from build123d import *

# Parameters (mm, degrees)
F0_R     = 6.35
F0_R_2   = 5.588
F1_DEPTH = 6.35
F0_R_3   = 0.638783
F0_R_4   = 1.905
F2_DEPTH = 5.969


with BuildPart() as f1:
    # F0 (on Top) → F1 (new body, symmetric)
    with BuildSketch(Plane.XY):
        Circle(F0_R)
        Circle(F0_R_2, mode=Mode.SUBTRACT)
    extrude(amount=F1_DEPTH, both=True)

    # F0 (on Top) → F2 (join, symmetric)
    with BuildSketch(Plane.XY):
        Circle(F0_R_2)
        with Locations((-2.271086, -3.125882)):
            Circle(F0_R_3, mode=Mode.SUBTRACT)
        Circle(F0_R_4, mode=Mode.SUBTRACT)
        with Locations((2.271086, -3.125882)):
            Circle(F0_R_3, mode=Mode.SUBTRACT)
        with Locations((-3.674694, 1.193981)):
            Circle(F0_R_3, mode=Mode.SUBTRACT)
        with Locations((0, 3.863802)):
            Circle(F0_R_3, mode=Mode.SUBTRACT)
        with Locations((3.674694, 1.193981)):
            Circle(F0_R_3, mode=Mode.SUBTRACT)
    extrude(amount=F2_DEPTH, both=True)


solid = f1.part
Verification items for the finished model (mm, model axes). A direction names the side the tool comes from. Coordinates: 2 decimals unless noted, no trailing zeros. Order: outer loops, then holes, each group sorted by start corner. A loop starts at its lowest first (then second) coordinate and runs counter-clockwise, first axis right, second up. Notation, with made-up numbers: M 85.25,-6 L 94.25,-6 A10 cw 94.25,1 Z; hole C 37.5,22 d1. An arc over 180 degrees is marked long. One line per item, written item: value. Start each with the question number.
Item 1: Mould release check, pull along X, two halves, no side actions. Record for faces 1 (the cylindrical face through (-1.38, -6.2, 0.09)), 2 (the cylindrical face through (2.88, -2.93, -0.08)), 3 (the flat face through (0, -6, 6.35)): released by +X, released by -X, zero draft, split by the parting line, or undercut.
Item 2: Gauge pin test, flat ends, axial feed: pin 1 (1.5 mm diameter, centred on y = -2.5, z = 2, fed in from -X); pin 2 (1.5 mm diameter, centred on x = -4, z = -2.5, fed in from +Y); pin 3 (2 mm diameter, centred on y = -1.5, z = 2, fed in from +X); pin 4 (4 mm diameter, centred on x = -5, y = 1.5, fed in from +Z). Record the tip position at first contact, or that the pin passes through.
Item 3: Scan lines: probe 1 along X at (y, z) = (1, 0.25); probe 2 along Y at (x, z) = (0, 6); probe 3 along Z at (x, y) = (1.5, -1.5). Record each from-to range of solid material in increasing order.
Item 4: Sectioned sample at B-B (x = 0). Enter the section's corners in (y, z) (3 decimals).
Item 5: Access from +Z, -Z, +X, -X, +Y, -Y to the whole of each face (thin tool, end or side, straight path). Record for faces 4 (the flat face through (2.4, 0.1, -5.969)), 5 (the flat face through (2.4, 0.1, 5.969)), 6 (the cylindrical face through (-3.085, 0.949, -0.084)).
Item 6: Sectioned sample at D-D (z = 3). Enter the section's corners in (x, y) (3 decimals), then the cut area to 3 significant figures.
Item 7: Sectioned sample at C-C (x = -3.25). Enter the section's corners in (y, z), then the cut area to 3 significant figures.
Item 8: Sectioned sample at A-A (y = 0). Enter the section's corners in (x, z) (3 decimals).
Conclusion:
1. face 1: split by the parting line
1. face 2: undercut
1. face 3: zero draft
2. pin 1: stops at x = -6.1
2. pin 2: stops at y = 5.46
2. pin 3: stops at x = 6.33
2. pin 4: stops at z = 6.35
3. probe 1: x = -6.27 to -4.28, -3.07 to -1.62, 1.62 to 3.07, 4.28 to 6.27
3. probe 2: y = -6.35 to -5.59, 5.59 to 6.35
3. probe 3: z = -5.97 to 5.97
4. outline: M -6.35,-6.35 L -5.588,-6.35 L -5.588,-5.969 L -1.905,-5.969 L -1.905,5.969 L -5.588,5.969 L -5.588,6.35 L -6.35,6.35 Z; M 1.905,-5.969 L 3.225,-5.969 L 3.225,5.969 L 1.905,5.969 Z; M 4.503,-5.969 L 5.588,-5.969 L 5.588,-6.35 L 6.35,-6.35 L 6.35,6.35 L 5.588,6.35 L 5.588,5.969 L 4.503,5.969 Z
5. face 4: -Z
5. face 5: +Z
5. face 6: +Z, -Z
6. outline: C 0,0 d12.7; hole C -3.675,1.194 d1.278; hole C -2.271,-3.126 d1.278; hole C 0,0 d3.81; hole C 0,3.864 d1.278; hole C 2.271,-3.126 d1.278; hole C 3.675,1.194 d1.278
6. area: 109 mm^2
7. outline: M -5.46,-6.35 L -4.55,-6.35 L -4.55,-5.97 L 0.72,-5.97 L 0.72,5.97 L -4.55,5.97 L -4.55,6.35 L -5.46,6.35 Z; M 1.67,-5.97 L 4.55,-5.97 L 4.55,-6.35 L 5.46,-6.35 L 5.46,6.35 L 4.55,6.35 L 4.55,5.97 L 1.67,5.97 Z
7. area: 120 mm^2
8. outline: M -6.35,-6.35 L -5.588,-6.35 L -5.588,-5.969 L -1.905,-5.969 L -1.905,5.969 L -5.588,5.969 L -5.588,6.35 L -6.35,6.35 Z; M 1.905,-5.969 L 5.588,-5.969 L 5.588,-6.35 L 6.35,-6.35 L 6.35,6.35 L 5.588,6.35 L 5.588,5.969 L 1.905,5.969 Z
